Check sheet for the modelled part. Datum: model origin and axes. Units: mm. A direction names the side the tool comes from. Give positions to 0.01 mm unless a question says otherwise; leave off trailing zeros. Order: outer loops, then holes, each group sorted by start corner. A loop starts at its lowest first (then second) coordinate and runs counter-clockwise, first axis right, second up.
```python
from build123d import *

# Parameters (mm, degrees)
F1_DEPTH       = 19
F1_DEPTH_BACK  = 19
F2_R           = 3
F3_T           = -2
F4_W           = 34
F4_H           = 26
F5_DEPTH       = 2
F6_R           = 11.5
F7_DEPTH       = 2
F9_D           = 3
F9_CSINK_D     = 6
F9_CSINK_ANGLE = 90
F11_D          = 3
F11_DEPTH      = 12
F12_R          = 10
F13_R          = 10
F14_R          = 10


with BuildPart() as f1:
    # F0 (on Right) → F1 (new body, two sides)
    with BuildSketch(Plane.YZ) as f1_sk:
        Polygon((0, 35), (0, 0), (30, 0), (30, 25), (10, 45), align=None)
    extrude(amount=F1_DEPTH)
    extrude(f1_sk.sketch, amount=-F1_DEPTH_BACK)

    # F2
    f2_edges = [f1.edges().sort_by_distance(p)[0] for p in [
        (0, 10, 45),
        (0, 0, 35),
        (0, 30, 25),
    ]]
    fillet(f2_edges, radius=F2_R)

    # F3
    f3_openings = [f1.faces().sort_by_distance(p)[0] for p in [
        (0, 15, 0),
    ]]
    offset(amount=F3_T, openings=f3_openings)

    # F4 (on Top) → F5 (join)
    with BuildSketch(Plane.XY):
        with BuildLine():
            Line((-29, 0), (29, 0))
            Line((29, 0), (29, 20))
            ThreePointArc((29, 20), (26.071068, 27.071068), (19, 30))
            Line((19, 30), (-17, 30))
            Line((-17, 30), (-29, 30))
            Line((-29, 30), (-29, 0))
        make_face()
        with Locations((0, 15)):
            Rectangle(F4_W, F4_H, mode=Mode.SUBTRACT)
    extrude(amount=-F5_DEPTH)

    # F6 (on face) → F7 (cut, through all)
    with BuildSketch(Plane(origin=(0, 27.5, 27.5), x_dir=(-1, 0, 0), z_dir=(0, 0.707107, 0.707107))):
        with Locations((0, 9.727922)):
            Circle(F6_R)
    extrude(amount=-F7_DEPTH, mode=Mode.SUBTRACT)

    # F9 (through all)
    with Locations(Plane.XY):
        with Locations((24.5, 15), (-24.5, 15)):
            CounterSinkHole(F9_D / 2, F9_CSINK_D / 2, counter_sink_angle=F9_CSINK_ANGLE)

    # F11
    with Locations(Plane.XZ):
        with Locations((0, 5)):
            Hole(F11_D / 2, depth=F11_DEPTH)

    # F12
    f12_edges = [f1.edges().sort_by_distance(p)[0] for p in [
        (29, 0, -1),
    ]]
    fillet(f12_edges, radius=F12_R)

    # F13
    f13_edges = [f1.edges().sort_by_distance(p)[0] for p in [
        (-29, 30, -1),
    ]]
    fillet(f13_edges, radius=F13_R)

    # F14
    f14_edges = [f1.edges().sort_by_distance(p)[0] for p in [
        (-29, 0, -1),
    ]]
    fillet(f14_edges, radius=F14_R)


solid = f1.part
```
(1) Go/stop test with flat-tipped pins: P1, Ø5, axis at x = 13, y = 14, coming from the +Z side; P2, Ø13, axis at y = 10.5, z = 18.5, coming from the -X side; P3, Ø1, axis at x = -5, z = 33.5, coming from the +Y side. Record where each tip stops, or that it passes through.
(2) Sectioned sample at D-D (y = 3). Enter the section's corners in (x, z).
(3) Sectioned sample at B-B (x = 9.5). Enter the section's corners in (y, z), plus the area to 3 significant figures.
(4) Thickness scan on L1, parallel to X at y = 15, z = -1.65; L2, parallel to X at y = 9, z = 27; L3, parallel to Y at x = -14, z = 15.5. Record the ranges inside material, lowest first.
(5) Release check for a two-part mould opening along Y. For faces 6 (the face through (0, 28, 11)), 7 (the face through (0, 29, -2)), 8 (the face through (0, 0, 16)) record: released by +Y, released by -Y, zero draft, split by the parting line, or undercut.
(6) Tool access check on faces 1 (the face through (21, 15, 0)), 2 (the face through (29, 15, -1)), 3 (the face through (-0.266, 9.967, 43.757)), 4 (the face through (-21, 15, 0)), 5 (the face through (11.57, 21.21, 30.96)). Record the directions out of +Z, -Z, +X, -X, +Y, -Y that give a thin tool (end or side, any length) a straight path to the whole face; none if there is none.
(7) Sectioned sample at C-C (x = 15.5). Enter the section's corners in (y, z), plus the area to 3 significant figures.
(8) Sectioned sample at A-A (z = 1). Enter the section's corners in (x, y), plus the area to 3 significant figures.
Values follow:
1. P1: stops at z = 43.36
1. P2: stops at x = -19
1. P3: stops at y = 2.03
2. outline: (-26.14, -2) - (-17, -2) - (-17, 35.17) - (17, 35.17) - (17, -2) - (26.14, -2) - (26.14, 0) - (19, 0) - (19, 38) - (-19, 38) - (-19, 0) - (-26.14, 0) - close
3. outline: (0, -2) - (2, -2) - (2, 33.76) arc R1 cw to (2.29, 34.46) - (9.29, 41.46) arc R1 cw to (10.71, 41.46) - (14.62, 37.55) - (16.04, 38.96) - (12.12, 42.88) arc R3 ccw to (7.88, 42.88) - (0.88, 35.88) arc R3 ccw to (0, 33.76) - close; (23.79, 28.38) - (27.71, 24.46) arc R1 cw to (28, 23.76) - (28, -2) - (30, -2) - (30, 23.76) arc R3 ccw to (29.12, 25.88) - (25.2, 29.8) - close
3. area: 178 mm2
4. L1: x = -29 to -26, -23 to -17, 17 to 23, 26 to 29
4. L2: x = -19 to -17, 17 to 19
4. L3: y = 0 to 2, 28 to 30
5. face 6: undercut
5. face 7: zero draft
5. face 8: released by -Y
6. face 1: +Z, +X, +Y, -Y
6. face 2: +Z, -Z, +X, +Y, -Y
6. face 3: +Z, +X, -X
6. face 4: +Z, -X, +Y, -Y
6. face 5: -Z
7. outline: (0, -2) - (2, -2) - (2, 33.76) arc R1 cw to (2.29, 34.46) - (9.29, 41.46) arc R1 cw to (10.71, 41.46) - (27.71, 24.46) arc R1 cw to (28, 23.76) - (28, -2) - (30, -2) - (30, 23.76) arc R3 ccw to (29.12, 25.88) - (12.12, 42.88) arc R3 ccw to (7.88, 42.88) - (0.88, 35.88) arc R3 ccw to (0, 33.76) - close
7. area: 203 mm2
8. outline: (-19, 0) - (19, 0) - (19, 30) - (-19, 30) - close; hole (-17, 2) - (17, 2) - (17, 28) - (-17, 28) - close
8. area: 256 mm2
